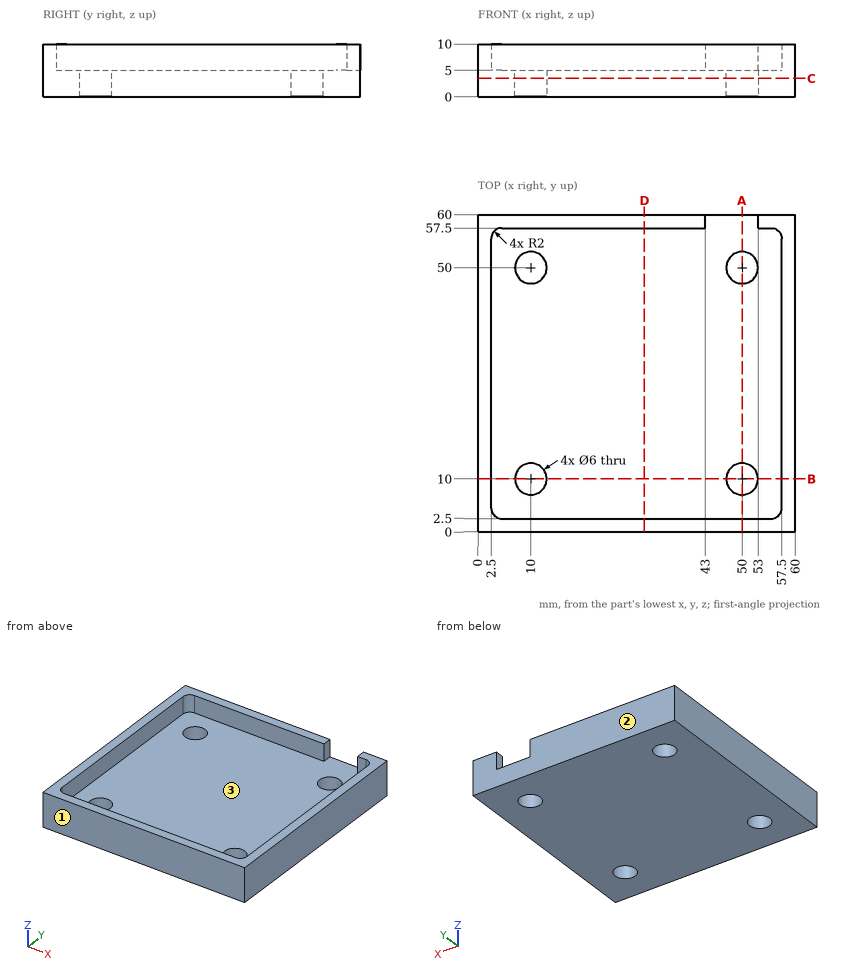
Geometry check sheet. Reference: drawing and pictorial views, mm from the part's lowest x, y, z. Round coordinates to 2 decimals unless told otherwise and drop trailing zeros. Order: outer loops, then holes, each group sorted by start corner. A loop starts at its lowest first (then second) coordinate and runs counter-clockwise, first axis right, second up. Notation, with made-up numbers: M 46.5,23 L 80.5,23 A5 ccw 80.5,27 Z; hole C 86,-40 d9. An arc over 180 degrees is marked long. Answer as CSV lines item,"result".
1) Sectioned sample at D-D on x = 31.5. Record the cut outline in (y, z).
Entries:
outline,"M 0,0 L 60,0 L 60,10 L 57.5,10 L 57.5,5 L 2.5,5 L 2.5,10 L 0,10 Z"
2) Sectioned sample at A-A on x = 50. Record the cut outline in (y, z).
Entries:
outline,"M 0,0 L 7,0 L 7,5 L 2.5,5 L 2.5,10 L 0,10 Z; M 13,0 L 47,0 L 47,5 L 13,5 Z; M 53,0 L 60,0 L 60,5 L 53,5 Z"
3) Sectioned sample at B-B on y = 10. Record the cut outline in (x, z), and give its area (3 significant figures).
Entries:
outline,"M 0,0 L 7,0 L 7,5 L 2.5,5 L 2.5,10 L 0,10 Z; M 13,0 L 47,0 L 47,5 L 13,5 Z; M 53,0 L 60,0 L 60,10 L 57.5,10 L 57.5,5 L 53,5 Z"
area,"265 mm2"
4) Thickness scan on probe 1 along Y at (x, z) = (10, 1.4); probe 2 along X at (y, z) = (55, 8.75). Record the ranges inside material, lowest first. Write a range as [from, to].
Entries:
probe 1,"[0, 7], [13, 47], [53, 60]"
probe 2,"[0, 2.5], [57.5, 60]"
5) Sectioned sample at C-C on z = 3.5. Record the cut outline in (x, y), and give its area (3 significant figures).
Entries:
outline,"M 0,0 L 60,0 L 60,60 L 0,60 Z; hole C 10,10 d6; hole C 10,50 d6; hole C 50,10 d6; hole C 50,50 d6"
area,"3,490 mm2"
6) Gauge pin test, flat ends, axial feed: pin 1 Ø7 at (x, y) = (50, 50) entering from +Z; pin 2 Ø5.5 at (x, y) = (10, 10) entering from -Z. Record the tip position at first contact, or that the pin passes through.
Entries:
pin 1,"z = 5"
pin 2,"through"
7) Mould release check, pull along Y, two halves, no side actions. Record for the marked faces 1, 2 and 3: +Y half, -Y half, draft (parallel to the pull), parting line (faces both ways), or undercut.
Entries:
face 1,"-Y half"
face 2,"+Y half"
face 3,"undercut"
